```python
from build123d import *

# Parameters (mm, degrees)
SKETCH_1_W          = 20
SKETCH_1_H          = 20
SKETCH_1_R          = 3
EXTRUDE_1_DEPTH     = 10
SKETCH_2_R          = 3
CUT_EXTRUDE_1_DEPTH = 30.298841179
CHAMFER_3_SIZE      = 0.5
CHAMFER_4_SIZE      = 0.2


with BuildPart() as part:
    # 草图1 → 凸台-拉伸1 (new body)
    with BuildSketch(Plane(origin=(0, 0, 0), x_dir=(1, 0, 0), z_dir=(0, 1, 0))):
        with Locations((8.932038835, -3.155339806)):
            Rectangle(SKETCH_1_W, SKETCH_1_H)
        with Locations(Location((5.432038835, -3.155339806, 0), (0, 0, 270))):
            Circle(SKETCH_1_R, mode=Mode.SUBTRACT)
    extrude(amount=EXTRUDE_1_DEPTH)

    # 草图2 → 切除-拉伸1 (cut, through all)
    with BuildSketch(Plane(origin=(0, 0, -6.844660194), x_dir=(-1, 0, 0), z_dir=(0, 0, -1))):
        with Locations((-12.432038835, 5)):
            Circle(SKETCH_2_R)
    extrude(amount=-CUT_EXTRUDE_1_DEPTH, mode=Mode.SUBTRACT)

    # 倒角3
    chamfer_3_edges = [part.edges().sort_by_distance(p)[0] for p in [
        (5.432038835, 0, 0.155339806),
        (5.432038835, 10, 0.155339806),
        (15.432038835, 5, 13.155339806),
        (15.432038835, 5, -6.844660194),
    ]]
    chamfer(chamfer_3_edges, length=CHAMFER_3_SIZE)

    # 倒角4
    chamfer_4_edges = [part.edges().sort_by_distance(p)[0] for p in [
        (18.932038835, 10, 3.155339806),
        (8.932038835, 10, -6.844660194),
        (-1.067961165, 10, 3.155339806),
        (8.932038835, 0, -6.844660194),
        (18.932038835, 0, 3.155339806),
        (8.932038835, 0, 13.155339806),
        (-1.067961165, 0, 3.155339806),
        (8.932038835, 10, 13.155339806),
        (-1.067961165, 5, -6.844660194),
        (18.932038835, 5, -6.844660194),
        (18.932038835, 5, 13.155339806),
        (-1.067961165, 5, 13.155339806),
    ]]
    chamfer(chamfer_4_edges, length=CHAMFER_4_SIZE)


solid = part.part
```
Check sheet for the modelled part. Datum: model origin and axes. Units: mm. Round coordinates to 2 decimals unless told otherwise and drop trailing zeros. Loops run counter-clockwise (first coordinate to the right, second up) from the corner with the lowest first, then second, coordinate; pieces in that order, holes last. Notation, with made-up numbers: M -23.5,-25.5 L 5.5,-25.5 A15 cw 5.5,-19.5 Z; hole C 88.25,32 d11. An arc over 180 degrees is marked long. Answer as a JSON object with one key per item and string values.
1. Section check A-A (y = 5). Record the boundary of the cut face in (x, z), plus the area to 3 significant figures.
Reply:
{"outline": "M -1.07,-6.64 L -0.87,-6.84 L 8.93,-6.84 L 9.43,-6.34 L 9.43,12.66 L 8.93,13.16 L -0.87,13.16 L -1.07,12.96 Z; M 15.43,-6.34 L 15.93,-6.84 L 18.73,-6.84 L 18.93,-6.64 L 18.93,12.96 L 18.73,13.16 L 15.93,13.16 L 15.43,12.66 Z; hole C 5.43,3.16 d6", "area": "251 mm²"}
2. Scan lines: line 1 (X direction, y = 2.5, z = 1.75); line 2 (X direction, y = 4.5, z = -1.75); line 3 (X direction, y = 4.75, z = 8.25). Record each from-to range of solid material in increasing order.
Reply:
{"line 1": "x = -1.07 to 2.78, 8.08 to 10.77, 14.09 to 18.93", "line 2": "x = -1.07 to 9.47, 15.39 to 18.93", "line 3": "x = -1.07 to 9.44, 15.42 to 18.93"}
3. Section check B-B (z = -2). Record the boundary of the cut face in (x, y), plus the area to 3 significant figures.
Reply:
{"outline": "M -1.07,0.2 L -0.87,0 L 18.73,0 L 18.93,0.2 L 18.93,9.8 L 18.73,10 L -0.87,10 L -1.07,9.8 Z; hole C 12.43,5 d6", "area": "172 mm²"}
4. Mould release check, pull along Z, two halves, no side actions. Record for faces 1 (the flat face through (7, 5, 13.155)), 2 (the flat face through (7, 5, -6.845)), 3 (the cylindrical face through (2.503, 4.937, 2.505)), 4 (the flat face through (-1.068, 5, 3)): pulls with the +Z half, pulls with the -Z half, needs draft (parallel to the pull), parting line crosses it, or undercut.
Reply:
{"face 1": "pulls with the +Z half", "face 2": "pulls with the -Z half", "face 3": "undercut", "face 4": "needs draft"}
5. Gauge pin test, flat end, axial feed: P1, Ø10, axis at x = 6, z = 3, coming from the -Y side. Record the tip position at first contact, or that the pin passes through.
Reply:
{"P1": "stops at y = 0"}
6. Section check C-C (y = 1). Record the boundary of the cut face in (x, z).
Reply:
{"outline": "M -1.07,-6.64 L -0.87,-6.84 L 18.73,-6.84 L 18.93,-6.64 L 18.93,12.96 L 18.73,13.16 L -0.87,13.16 L -1.07,12.96 Z; hole C 5.43,3.16 d6"}
7. Section check D-D (y = 3.75). State how many separate pieces and enclosed holes the cut face has, plus the area to 3 significant figures.
Reply:
{"separate pieces": "2", "enclosed holes": "1", "area": "262 mm²"}
